```python
from build123d import *

# Parameters (mm, degrees)
SKETCH1_W                                  = 609.6
SKETCH1_H                                  = 609.6
BOSS_EXTRUDE1_DEPTH                        = 76.2
SKETCH2_W                                  = 457.2
SKETCH2_H                                  = 203.2
CUT_EXTRUDE1_DEPTH                         = 76.2
SKETCH3_R                                  = 12.7
CUT_EXTRUDE2_DEPTH                         = 38.1
MIRROR1_AT_THE_SECOND_PLANE_COPY_1_SKETC_R = 12.7
MIRROR1_AT_THE_SECOND_PLANE_COPY_1_DEPTH   = 38.1
SKETCH6_R                                  = 74.93
CUT_EXTRUDE3_DEPTH                         = 6.35
FILLET1_R                                  = 2.54
SKETCH7_R                                  = 4.4958
CUT_EXTRUDE4_DEPTH                         = 20
CIRPATTERN1_COUNT                          = 4
FILLET2_R                                  = 10


with BuildPart() as part:
    # Sketch1 → Boss-Extrude1 (new body)
    with BuildSketch(Plane(origin=(0, 0, 0), x_dir=(1, 0, 0), z_dir=(0, 1, 0))):
        Rectangle(SKETCH1_W, SKETCH1_H)
    extrude(amount=BOSS_EXTRUDE1_DEPTH)

    # Sketch2 → Cut-Extrude1 (cut)
    with BuildSketch(Plane(origin=(0, 76.2, 0), x_dir=(1, 0, 0), z_dir=(0, 1, 0))):
        with Locations((0, -203.2)):
            Rectangle(SKETCH2_W, SKETCH2_H)
        with Locations((0, 203.2)):
            Rectangle(SKETCH2_W, SKETCH2_H)
    extrude(amount=-CUT_EXTRUDE1_DEPTH, mode=Mode.SUBTRACT)

    # Sketch3 → Cut-Extrude2 (cut)
    with BuildSketch(Plane(origin=(0, 76.2, 0), x_dir=(1, 0, 0), z_dir=(0, 1, 0))):
        with Locations(Location((-266.7, 266.7, 0), (0, 0, 270))):
            Circle(SKETCH3_R)
    cut_extrude2 = extrude(amount=-CUT_EXTRUDE2_DEPTH, mode=Mode.SUBTRACT)

    # Mirror1: Cut-Extrude2 across plane
    add(cut_extrude2.mirror(Plane(origin=(0, 0, 0), x_dir=(0, 0, 1), z_dir=(1, 0, 0))), mode=Mode.SUBTRACT)

    # Mirror1 at the second plane: Cut-Extrude2 across plane
    add(cut_extrude2.mirror(Plane.XY), mode=Mode.SUBTRACT)

    # Mirror1 at the second plane copy 1 sketc → Mirror1 at the second plane copy 1 (cut)
    with BuildSketch(Plane(origin=(0, 76.2, 0), x_dir=(-1, 0, 0), z_dir=(0, 1, 0))):
        with Locations(Location((-266.7, 266.7, 0), (0, 0, 270))):
            Circle(MIRROR1_AT_THE_SECOND_PLANE_COPY_1_SKETC_R)
    extrude(amount=-MIRROR1_AT_THE_SECOND_PLANE_COPY_1_DEPTH, mode=Mode.SUBTRACT)

    # Sketch6 → Cut-Extrude3 (cut)
    with BuildSketch(Plane.XZ):
        with Locations(Location((0, 0, 0), (0, 0, 270))):
            Circle(SKETCH6_R)
    extrude(amount=-CUT_EXTRUDE3_DEPTH, mode=Mode.SUBTRACT)

    # Fillet1
    fillet1_edges = [part.edges().sort_by_distance(p)[0] for p in [
        (0, 0, 74.93),
    ]]
    fillet(fillet1_edges, radius=FILLET1_R)

    # Sketch7 → Cut-Extrude4 (cut)
    with BuildSketch(Plane.XZ):
        with Locations(Location((0, 66, 0), (0, 0, 270))):
            Circle(SKETCH7_R)
    cut_extrude4 = extrude(amount=-CUT_EXTRUDE4_DEPTH, mode=Mode.SUBTRACT)

    # CirPattern1: Cut-Extrude4 ×4 about axis
    cirpattern1_axis = Axis((0, 0, 0), (0, 1, 0))
    for i in range(1, CIRPATTERN1_COUNT):
        add(cut_extrude4.rotate(cirpattern1_axis, i * 360 / CIRPATTERN1_COUNT), mode=Mode.SUBTRACT)

    # Fillet2
    fillet2_edges = [part.edges().sort_by_distance(p)[0] for p in [
        (-304.8, 76.2, 0),
        (-228.6, 0, 203.2),
        (0, 0, 101.6),
        (228.6, 0, 203.2),
        (-228.6, 76.2, 203.2),
        (228.6, 76.2, 203.2),
        (0, 76.2, 101.6),
        (-228.6, 0, -203.2),
        (228.6, 0, -203.2),
        (0, 0, -101.6),
        (-228.6, 76.2, -203.2),
        (0, 76.2, -101.6),
        (228.6, 76.2, -203.2),
        (304.8, 76.2, 0),
        (-304.8, 0, 0),
        (304.8, 0, 0),
    ]]
    fillet(fillet2_edges, radius=FILLET2_R)


solid = part.part
```
Model file for the job. Use its own axes, mm. A direction names the side the tool comes from. Round coordinates to 2 decimals unless told otherwise and drop trailing zeros. Write each loop counter-clockwise with the first axis right and the second up, starting at its lowest first coordinate (ties: lowest second). Pieces come first, ordered by that corner, then holes. Notation, with made-up numbers: M 82,44 L 122,44 A21 cw 122,62 Z; hole C -3.75,-37.5 d2. An arc over 180 degrees is marked long. Put each result on its own line as item: value.
Item 1: Probe L1, parallel to Z at x = 266.7, y = 53; L2, parallel to X at y = 33, z = -119; L3, parallel to X at y = 72, z = 150. List the from-to ranges inside material, lowest first. Write a range as from..to.
Responses:
L1: -304.8..-279.4, -254..254, 279.4..304.8
L2: -304.8..-228.6, 228.6..304.8
L3: -302.95..-230.45, 230.45..302.95
Item 2: Flat gauge pins, fed straight in: P1, Ø4.5, axis at x = -1, z = -67, coming from the -Y side; P2, Ø7.5, axis at x = -272.5, z = -271.5, coming from the +Y side; P3, Ø7, axis at x = 2, z = 66, coming from the -Y side. Where does each tip first touch, or does it go through?
Responses:
P1: y = 20
P2: y = 38.1
P3: y = 6.35
Item 3: Cut at A-A (z = -171.5). List the corners of the cut face in (x, y), and give its area (3 significant figures).
Responses:
outline: M -304.8,10 A10 ccw -294.8,0 L -238.6,0 A10 ccw -228.6,10 L -228.6,66.2 A10 ccw -238.6,76.2 L -294.8,76.2 A10 ccw -304.8,66.2 Z; M 228.6,10 A10 ccw 238.6,0 L 294.8,0 A10 ccw 304.8,10 L 304.8,66.2 A10 ccw 294.8,76.2 L 238.6,76.2 A10 ccw 228.6,66.2 Z
area: 11,400 mm²
Item 4: Cut at B-B (x = 266.7). List the corners of the cut face in (y, z), and give its area (3 significant figures).
Responses:
outline: M 0,-304.8 L 76.2,-304.8 L 76.2,-279.4 L 38.1,-279.4 L 38.1,-254 L 76.2,-254 L 76.2,254 L 38.1,254 L 38.1,279.4 L 76.2,279.4 L 76.2,304.8 L 0,304.8 Z
area: 44,500 mm²
Item 5: Cut at D-D (x = 136). List the corners of the cut face in (y, z), and give its area (3 significant figures).
Responses:
outline: M 0,-91.6 A10 ccw 10,-101.6 L 66.2,-101.6 A10 ccw 76.2,-91.6 L 76.2,91.6 A10 ccw 66.2,101.6 L 10,101.6 A10 ccw 0,91.6 Z
area: 15,400 mm²
Item 6: Cut at C-C (z = -266.7). List the corners of the cut face in (x, y), and give its area (3 significant figures).
Responses:
outline: M -304.8,10 A10 ccw -294.8,0 L -238.6,0 A10 ccw -228.6,10 L -228.6,66.2 A10 ccw -238.6,76.2 L -254,76.2 L -254,38.1 L -279.4,38.1 L -279.4,76.2 L -294.8,76.2 A10 ccw -304.8,66.2 Z; M 228.6,10 A10 ccw 238.6,0 L 294.8,0 A10 ccw 304.8,10 L 304.8,66.2 A10 ccw 294.8,76.2 L 279.4,76.2 L 279.4,38.1 L 254,38.1 L 254,76.2 L 238.6,76.2 A10 ccw 228.6,66.2 Z
area: 9,510 mm²
Item 7: Tool access for faces 1 (the flat face through (-3, 38, 101.6)), 2 (the flat face through (267, 38.1, -267)), 3 (the flat face through (1, 6.35, 1)), 4 (the flat face through (228.6, 38, -202)): list every direction of +Z, -Z, +X, -X, +Y, -Y with a clear straight run to the whole face (end or side of a thin tool).
Responses:
face 1: +Z, +Y, -Y
face 2: +Y
face 3: -Y
face 4: -Z, +Y, -Y
Item 8: Mould opens along X. For faces 5 (the flat face through (266, 38, 304.8)), 6 (the cylindrical face through (255.991, 57.417, -259.873)), 7 (the flat face through (-304.8, 38, 4)) say: +X half, -X half, draft (parallel to the pull), parting line (faces both ways), or undercut.
Responses:
face 5: draft
face 6: undercut
face 7: -X half
